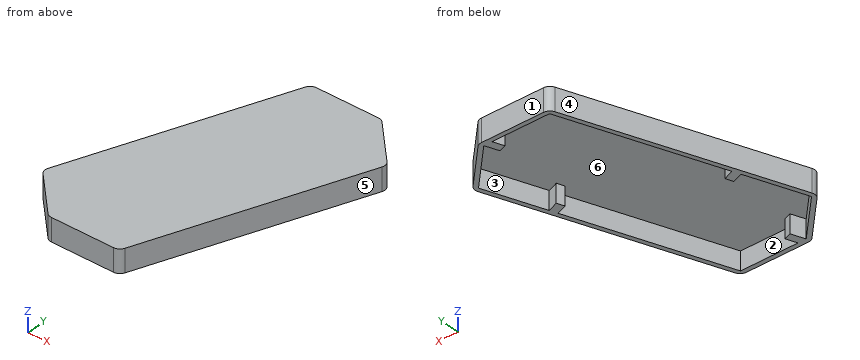
Autodesk Inventor part; units mm, degrees
ref_plane "YZ Plane" through (0, 0, 0) normal (1, 0, 0) x (0, 1, 0)
ref_plane "XZ Plane" through (0, 0, 0) normal (0, 1, 0) x (-1, 0, 0)
ref_plane "XY Plane" through (0, 0, 0) normal (0, 0, 1) x (1, 0, 0)
sketch "TopProfile" plane through (0, 0, 0) normal (0, 0, 1) x (1, 0, 0)
  line L0 (22.417, 108.5547) -> (40.2604, 90.5219)
  line L1 (-6.7187, 108.5547) -> (22.417, 108.5547)
  line L2 (-6.7187, 108.5547) -> (-40.2084, 18.0328)
  line L3 (40.2604, 90.5219) -> (6.7706, 0)
  line L4 (-22.3651, 0) -> (6.7706, 0)
  line L5 (-40.2084, 18.0328) -> (-22.3651, 0)
  line L6 (-35.2804, 13.0524) -> (0.052, 108.5547) construction
  line L7 (0.052, 108.5547) -> (35.3323, 95.5023) construction
  line L8 (35.3323, 95.5023) -> (0, 0) construction
  line L9 (0, 0) -> (-35.2804, 13.0524) construction
  line L10 (-56.3022, 0) -> (56.3541, 0) construction
  line L11 (-38.1479, 18.4782) -> (-21.6231, 1.778)
  line L12 (-21.6231, 1.778) -> (5.5327, 1.778)
  line L13 (5.5327, 1.778) -> (38.1998, 90.0765)
  line L14 (38.1998, 90.0765) -> (21.6751, 106.7767)
  line L15 (21.6751, 106.7767) -> (-5.4807, 106.7767)
  line L16 (-5.4807, 106.7767) -> (-38.1479, 18.4782)
  line L17 (-29.3346, 42.3002) -> (-28.233, 45.278)
  line L18 (-28.233, 45.278) -> (-23.945, 43.6916)
  line L19 (-23.945, 43.6916) -> (-25.0467, 40.7138)
  line L20 (-25.0467, 40.7138) -> (-29.3346, 42.3002)
  line L21 (25.0986, 67.8409) -> (29.3866, 66.2545)
  line L22 (29.3866, 66.2545) -> (28.2849, 63.2768)
  line L23 (28.2849, 63.2768) -> (23.997, 64.8632)
  line L24 (23.997, 64.8632) -> (25.0986, 67.8409)
  line L25 (16.6726, 102.4057) -> (19.6504, 101.304)
  line L26 (19.6504, 101.304) -> (21.6751, 106.7767)
  line L27 (21.6751, 106.7767) -> (18.6973, 107.8784)
  line L28 (18.6973, 107.8784) -> (16.6726, 102.4057)
  line L29 (-19.5984, 7.2507) -> (-16.6207, 6.149)
  line L30 (-16.6207, 6.149) -> (-18.6454, 0.6763)
  line L31 (-18.6454, 0.6763) -> (-21.6231, 1.778)
  line L32 (-21.6231, 1.778) -> (-19.5984, 7.2507)
  point P0 (-18.2378, 1.778)
  point P1 (18.2897, 106.7767)
  dimension "d0" = 29.1357
  dimension "d2" = 69.697
  dimension "d3" = 25
  dimension "d4" = 25
  dimension "d5" = 101.8286
  dimension "d6" = 37.6174
  dimension "d7" = 25.3686
  dimension "d8" = 1.778
  dimension "d17" = 3.175
  dimension "d18" = 25.4
  dimension "d19" = 25.4
extrude "CapFeature" add sketch "TopProfile" along normal blind 1.778 contours L0 L3 L4 L5 L2 L1 | L16 L20 L19 L18 L15 L28 L25 L26 L14 L13 L21 L24 L23 L12 L30 L29 L32 L11 | L32 L29 L30 L12 | L12 L30 L31 | L16 L18 L19 L20 | L23 L24 L21 L13 | L28 L27 L15 | L15 L26 L25 L28
extrude "WallsFeature" add sketch "TopProfile" against normal blind 7.62 contours L0 L3 L4 L5 L2 L1 | L32 L29 L30 L12 | L12 L30 L31 | L16 L18 L19 L20 | L23 L24 L21 L13 | L28 L27 L15 | L15 L26 L25 L28
fillet "SideFilletsFeature" radius 3.175 6 edges at (-22.3651, 0, -2.921) (-40.2084, 18.0328, -2.921) (6.7706, 0, -2.921) (40.2604, 90.5219, -2.921) (22.417, 108.5547, -2.921) (-6.7187, 108.5547, -2.921)
equation "\"d19\" = d18"
properties part number "switchback-pickup-cover-8"
Geometry: final body of the model. Coordinates: model frame, mm. Face numbers are marked on the shaded views. A direction names the side the tool comes from. Give positions to 0.01 mm unless a question says otherwise; leave off trailing zeros. Write each loop counter-clockwise with the first axis right and the second up, starting at its lowest first coordinate (ties: lowest second). Pieces come first, ordered by that corner, then holes.
1. Line query: probe 1 along Z at (x, y) = (18, 54.5); probe 2 along X at (y, z) = (72, -6); probe 3 along X at (y, z) = (61, -1.25). Output: solid intervals per line, ascending.
2. Section query C-C, the plane x = 11.5. Return loops of the section in (y, z).
3. Section query A-A, the plane y = 22. Return loops of the section in (x, z), then the cut area to 3 significant figures.
4. Pin query (flat end, axial travel): P1, Ø1, axis at y = 18, z = -4.5, coming from the +X side; P2, Ø2, axis at x = 25, z = -6, coming from the +Y side; P3, Ø5, axis at x = -24, z = -6, coming from the -Y side. Return the tip coordinate at first contact, or that it passes through.
5. Reachability of the marked faces 5 and 6 from +Z, -Z, +X, -X, +Y, -Y: full face, straight path, thin tool, end or side. Return the list, or none.
6. Draft query along X for the marked faces 1, 2, 3 and 4. Return one class per face: released by +X, released by -X, zero draft, split by the parting line, or undercut.
Computed:
1. probe 1: z = 0 to 1.78
1. probe 2: x = -20.24 to -18.35, 31.51 to 33.41
1. probe 3: x = -24.31 to -22.42, 27.44 to 29.34
2. outline: (12.78, -7.62) - (17.91, -7.62) - (17.91, 0) - (106.78, 0) - (106.78, -7.62) - (108.55, -7.62) - (108.55, 1.78) - (12.78, 1.78) - close
3. outline: (-38.74, -7.62) - (-36.84, -7.62) - (-36.84, 0) - (13.01, 0) - (13.01, -7.62) - (14.91, -7.62) - (14.91, 1.78) - (-38.74, 1.78) - close
3. area: 124 mm2
4. P1: stops at x = 13.61
4. P2: stops at y = 106.95
4. P3: stops at y = 0.03
5. face 5: +Z, -Z, +X, -Y
5. face 6: -Z
6. face 1: zero draft
6. face 2: undercut
6. face 3: undercut
6. face 4: released by -X
